from build123d import *

# Parameters (mm, degrees)
BOSS_EXTRUDE1_DEPTH      = 37.5
BOSS_EXTRUDE1_DEPTH_BACK = 37.5
SKETCH1_W                = 20
SKETCH1_H                = 10
SKETCH3_W                = 20
SKETCH3_H                = 5
BOSS_EXTRUDE2_DEPTH      = 20
FILLET1_R                = 10
SKETCH4_R                = 2.75
CUT_EXTRUDE1_DEPTH       = 59.84301148
FILLET1_OF_MIRROR3_R     = 10
CHAMFER1_SIZE            = 8.660254038
CHAMFER1_SIZE_2          = 5


# Some blends are built 0.0001 mm under size
with BuildPart() as part:
    # Sketch1 → Boss-Extrude1 (new, two sides: drawn at the far end of the back side and taken through both)
    with BuildSketch(Plane.XY.offset(-BOSS_EXTRUDE1_DEPTH_BACK)):
        Rectangle(SKETCH1_W, SKETCH1_H)
    extrude(amount=BOSS_EXTRUDE1_DEPTH + BOSS_EXTRUDE1_DEPTH_BACK)

    # Sketch3 → Boss-Extrude2 (add)
    with BuildSketch(Plane(origin=(0, 0, -37.5), x_dir=(-1, 0, 0), z_dir=(0, 0, -1))):
        Rectangle(SKETCH3_W, SKETCH3_H)
    boss_extrude2 = extrude(amount=BOSS_EXTRUDE2_DEPTH)

    # Fillet1
    fillet1_edges = [part.edges().sort_by_distance(p)[0] for p in [
        (-10, 0, -57.5),
        (10, 0, -57.5),
    ]]
    fillet(fillet1_edges, radius=FILLET1_R - 0.0001)  # a hair under: the kernel refuses the full size

    # Sketch4 → Cut-Extrude1 (cut, through all)
    with BuildSketch(Plane(origin=(0, 2.5, 0), x_dir=(1, 0, 0), z_dir=(0, 1, 0))):
        with Locations(Location((0, 47.5, 0), (0, 0, 270))):
            Circle(SKETCH4_R)
    cut_extrude1 = extrude(amount=-CUT_EXTRUDE1_DEPTH, mode=Mode.SUBTRACT)

    # Mirror3: Boss-Extrude2, Cut-Extrude1 across plane
    add(boss_extrude2.mirror(Plane.XY))
    add(cut_extrude1.mirror(Plane.XY), mode=Mode.SUBTRACT)

    # Fillet1 of Mirror3
    fillet1_of_mirror3_edges = [part.edges().sort_by_distance(p)[0] for p in [
        (-10, 0, 57.5),
        (10, 0, 57.5),
    ]]
    fillet(fillet1_of_mirror3_edges, radius=FILLET1_OF_MIRROR3_R - 0.0001)  # a hair under: the kernel refuses the full size

    # Chamfer1
    # the kernel refuses this chamfer: 8.660254038, 5 mm, written as the material it takes off along each edge
    with BuildSketch(Plane(origin=(32.404819853, 5, -37.5), x_dir=(0, 0.019326765612700598, 0.9998132206222078), z_dir=(-1, 0, 0))) as chamfer1_piece_1_section:
        Polygon((CHAMFER1_SIZE * 0.999813220604, -CHAMFER1_SIZE * 0.0193267656124), (-CHAMFER1_SIZE_2 * 0.0193267656127, -CHAMFER1_SIZE_2 * 0.999813220622), (0, 0), align=None)
    chamfer1_piece_1 = extrude(amount=64.809639706, mode=Mode.PRIVATE)
    chamfer1_piece_1 = split(chamfer1_piece_1, bisect_by=Plane(origin=(0, 2.5, -34.039331058), z_dir=(0, 1, 0)), keep=Keep.TOP, mode=Mode.PRIVATE)
    add(chamfer1_piece_1, mode=Mode.SUBTRACT)
    with BuildSketch(Plane(origin=(-32.404819853, -5, -37.5), x_dir=(0, -0.019326765612700598, 0.9998132206222078), z_dir=(1, 0, 0))) as chamfer1_piece_2_section:
        Polygon((CHAMFER1_SIZE * 0.999813220604, -CHAMFER1_SIZE * 0.0193267656124), (-CHAMFER1_SIZE_2 * 0.0193267656127, -CHAMFER1_SIZE_2 * 0.999813220622), (0, 0), align=None)
    chamfer1_piece_2 = extrude(amount=64.809639706, mode=Mode.PRIVATE)
    chamfer1_piece_2 = split(chamfer1_piece_2, bisect_by=Plane(origin=(0, -2.5, -34.039331058), z_dir=(0, -1, 0)), keep=Keep.TOP, mode=Mode.PRIVATE)
    add(chamfer1_piece_2, mode=Mode.SUBTRACT)
    with BuildSketch(Plane(origin=(-32.404819853, -5, 37.5), x_dir=(0, 0.999813220622208, 0.019326765612700494), z_dir=(1, 0, 0))) as chamfer1_piece_3_section:
        Polygon((CHAMFER1_SIZE * 0.999813220604, -CHAMFER1_SIZE * 0.0193267656124), (-CHAMFER1_SIZE_2 * 0.0193267656127, -CHAMFER1_SIZE_2 * 0.999813220622), (0, 0), align=None)
    chamfer1_piece_3 = extrude(amount=64.809639706, mode=Mode.PRIVATE)
    chamfer1_piece_3 = split(chamfer1_piece_3, bisect_by=Plane(origin=(0, 2.5, 37.476500167), z_dir=(0, 1, 0)), keep=Keep.TOP, mode=Mode.PRIVATE)
    add(chamfer1_piece_3, mode=Mode.SUBTRACT)
    with BuildSketch(Plane(origin=(-32.404819853, -5, 37.5), x_dir=(0, 0.999813220622208, 0.019326765612700494), z_dir=(1, 0, 0))) as chamfer1_piece_4_section:
        Polygon((CHAMFER1_SIZE * 0.999813220604, -CHAMFER1_SIZE * 0.0193267656124), (-CHAMFER1_SIZE_2 * 0.0193267656127, -CHAMFER1_SIZE_2 * 0.999813220622), (0, 0), align=None)
    chamfer1_piece_4 = extrude(amount=64.809639706, mode=Mode.PRIVATE)
    chamfer1_piece_4 = split(chamfer1_piece_4, bisect_by=Plane(origin=(0, -2.5, 35.327003025), z_dir=(0, -1, 0)), keep=Keep.TOP, mode=Mode.PRIVATE)
    add(chamfer1_piece_4, mode=Mode.SUBTRACT)
    with BuildSketch(Plane(origin=(32.404819853, 5, 37.5), x_dir=(0, -0.999813220622208, 0.019326765612700494), z_dir=(-1, 0, 0))) as chamfer1_piece_5_section:
        Polygon((CHAMFER1_SIZE * 0.999813220604, -CHAMFER1_SIZE * 0.0193267656124), (-CHAMFER1_SIZE_2 * 0.0193267656127, -CHAMFER1_SIZE_2 * 0.999813220622), (0, 0), align=None)
    chamfer1_piece_5 = extrude(amount=64.809639706, mode=Mode.PRIVATE)
    chamfer1_piece_5 = split(chamfer1_piece_5, bisect_by=Plane(origin=(0, -2.5, 37.476500167), z_dir=(0, -1, 0)), keep=Keep.TOP, mode=Mode.PRIVATE)
    add(chamfer1_piece_5, mode=Mode.SUBTRACT)
    with BuildSketch(Plane(origin=(32.404819853, 5, 37.5), x_dir=(0, -0.999813220622208, 0.019326765612700494), z_dir=(-1, 0, 0))) as chamfer1_piece_6_section:
        Polygon((CHAMFER1_SIZE * 0.999813220604, -CHAMFER1_SIZE * 0.0193267656124), (-CHAMFER1_SIZE_2 * 0.0193267656127, -CHAMFER1_SIZE_2 * 0.999813220622), (0, 0), align=None)
    chamfer1_piece_6 = extrude(amount=64.809639706, mode=Mode.PRIVATE)
    chamfer1_piece_6 = split(chamfer1_piece_6, bisect_by=Plane(origin=(0, 2.5, 35.327003025), z_dir=(0, 1, 0)), keep=Keep.TOP, mode=Mode.PRIVATE)
    add(chamfer1_piece_6, mode=Mode.SUBTRACT)


solid = part.part
Could you check a few things on this model? Use its own coordinates, in mm. A direction names the side the tool comes from. Give positions to 0.01 mm unless a question says otherwise; leave off trailing zeros. Order: outer loops, then holes, each group sorted by start corner. A loop starts at its lowest first (then second) coordinate and runs counter-clockwise, first axis right, second up.
1. Suppose I cut it at D-D (x = -8.5). List the corners of the cut face in (y, z) for me.
2. Suppose I cut it at B-B (x = 6). List the corners of the cut face in (y, z) for me.
3. We'd pull the mould along X, two halves only. Please class faces 5 (the cylindrical face through (-7.15, 0.04, 54.49)), 6 (the cylindrical face through (0.121, 0.035, -50.247)), 7 (the flat face through (0, 2.5, -42)): pulls with the +X half, pulls with the -X half, needs draft (parallel to the pull), parting line crosses it, or undercut.
4. Suppose I cut it at C-C (z = 42.5). List the corners of the cut face in (x, y) for me.
5. Suppose I cut it at A-A (y = 1.5). Give the number of separate pieces and of enclosed holes in the cut face, plus the area to 3 significant figures.
6. Will these pins go through, and if not, where does the flat tip stop? P1, Ø1, axis at x = -6.5, y = 1, coming from the -Z side; P2, Ø5, axis at x = -4, y = -0.5, coming from the +Z side; P3, Ø10, axis at x = 4.5, z = 46.5, coming from the +Y side.
7. For faces 1 (the flat face through (0, -2.5, -42)), 2 (the cylindrical face through (0.121, 0.035, 50.247)), 3 (the flat face through (0, -2.5, 43)), 4 (the flat face through (0, 2.5, 43)), which set-ups out of +Z, -Z, +X, -X, +Y, -Y let a thin tool reach every point of the face, with its end or its side?
8. I need wall thicknesses on L1, parallel to X at y = 0, z = -47.5; L2, parallel to Z at x = -2.5, y = -0.5; L3, parallel to Z at x = -2, y = -1.75. Which ranges of each line are inside material? Lowest first, please.
Solved:
1. outline: (-5, -28.84) - (-2.5, -33.17) - (-2.5, -52.77) - (2.5, -52.77) - (2.5, -33.17) - (5, -28.84) - (5, 32.5) - (2.5, 33.94) - (2.5, 52.77) - (-2.5, 52.77) - (-2.5, 33.94) - (-5, 32.5) - close
2. outline: (-5, -28.84) - (-2.5, -33.17) - (-2.5, -55.5) - (2.5, -55.5) - (2.5, -33.17) - (5, -28.84) - (5, 32.5) - (2.5, 33.94) - (2.5, 55.5) - (-2.5, 55.5) - (-2.5, 33.94) - (-5, 32.5) - close
3. face 5: pulls with the -X half
3. face 6: undercut
3. face 7: needs draft
4. outline: (-10, -2.5) - (10, -2.5) - (10, 2.5) - (-10, 2.5) - close
5. separate pieces: 1
5. enclosed holes: 2
5. area: 2,170 mm2
6. P1: stops at z = -55.5
6. P2: stops at z = 57.39
6. P3: stops at y = 2.5
7. face 1: -Z, +X, -X, -Y
7. face 2: +Y, -Y
7. face 3: +Z, +X, -X, -Y
7. face 4: +Z, +X, -X, +Y
8. L1: x = -10 to -2.75, 2.75 to 10
8. L2: z = -57.18 to -48.65, -46.35 to 46.35, 48.65 to 57.18
8. L3: z = -57.3 to -49.39, -45.61 to 45.61, 49.39 to 57.3
